Check sheet for the drawn part. Datum: minimum x, y, z corner. Units: mm. Coordinates: 2 decimals unless noted, no trailing zeros. Loops run counter-clockwise (first coordinate to the right, second up) from the corner with the lowest first, then second, coordinate; pieces in that order, holes last. Notation, with made-up numbers: (76, 31) - (130, 31) arc R31 ccw to (130, 66) - close; hole circle Ø6 at (-8, 48). An arc over 180 degrees is marked (long way). Answer as CSV lines item,"result". Start each with the question number.
1. Gauge pin test, flat ends, axial feed: P1, Ø2, axis at y = 8.5, z = 129.5, coming from the -X side; P2, Ø10, axis at x = 498.5, z = 28.5, coming from the -Y side; P3, Ø1, axis at y = 7, z = 34, coming from the -X side; P4, Ø10, axis at y = 5, z = 116, coming from the -X side (3 decimals). Record the tip position at first contact, or that the pin passes through.
2. Cross-section at A-A (y = 24). Enter the section's corners in (x, z), plus the area to 3 significant figures.
3. Cross-section at B-B (x = 750). Enter the section's corners in (y, z).
4. Material ranges on line 1 (Z direction, x = 1450, y = 24); line 2 (X direction, y = 43, z = 91); line 3 (X direction, y = 28, z = 86.5), recorded low to high. Write a range as [from, to].
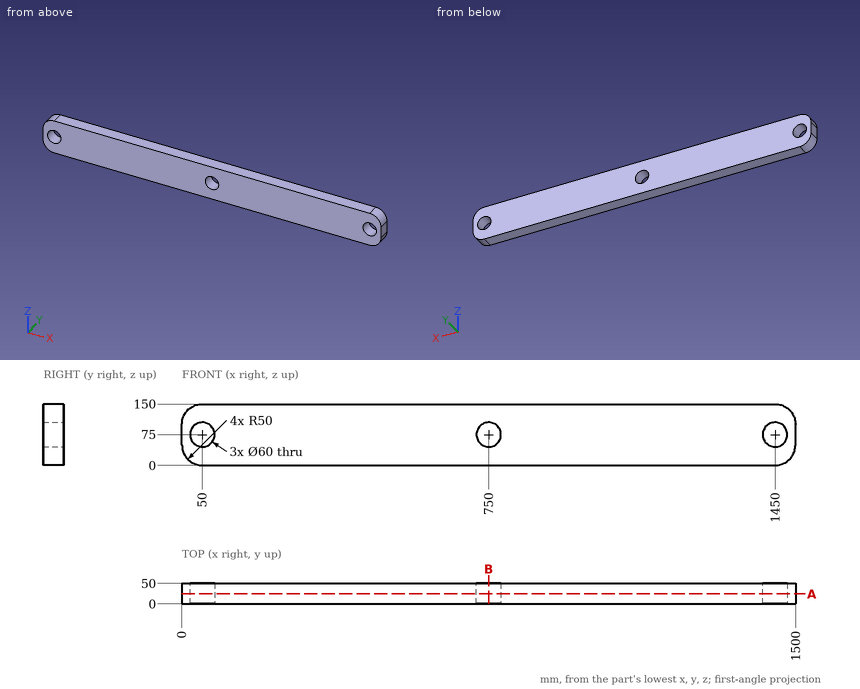
Values follow:
1,P1,"stops at x = 8.92"
1,P2,"stops at y = 0"
1,P3,"stops at x = 2.46"
1,P4,"stops at x = 1.225"
2,outline,"(0, 50) arc R50 ccw to (50, 0) - (1450, 0) arc R50 ccw to (1500, 50) - (1500, 100) arc R50 ccw to (1450, 150) - (50, 150) arc R50 ccw to (0, 100) - close; hole circle Ø60 at (50, 75); hole circle Ø60 at (750, 75); hole circle Ø60 at (1450, 75)"
2,area,"214,000 mm²"
3,outline,"(0, 0) - (50, 0) - (50, 45) - (0, 45) - close; (0, 105) - (50, 105) - (50, 150) - (0, 150) - close"
4,line 1,"z = [0, 45], [105, 150]"
4,line 2,"x = [0, 24.62], [75.38, 724.62], [775.38, 1424.62], [1475.38, 1500]"
4,line 3,"x = [0, 22.29], [77.71, 722.29], [777.71, 1422.29], [1477.71, 1500]"
